```python
from build123d import *

# Parameters (mm, degrees)
F0_R        = 31.3722800925
F1_DEPTH    = 2.4
F0_R_2      = 27.0541255518
F2_DEPTH    = 14.1
F3_T1_DEPTH = 394.7097038856


# Not quite as in the source:
# - a fillet or chamfer that OpenCascade refuses, or shapes differently, is made with other operations: its cross-section is extruded or revolved along the edge and cut away or added


with BuildPart() as f1:
    # F0 (on Front) → F1 (new body)
    with BuildSketch(Plane.XZ):
        Polygon((76.1774070561, 60.170147568), (-76.1774070561, 60.170147568), (-76.1774070561, 34.1583490372), (-76.1774070561, -34.1583490372), (-76.1774070561, -60.170147568), (76.1774070561, -60.170147568), (76.1774070561, -34.1583490372), (76.1774070561, 34.1583490372), align=None)
        Circle(F0_R, mode=Mode.SUBTRACT)
    extrude(amount=F1_DEPTH)

    # F0 (on Front) → F2 (join)
    with BuildSketch(Plane.XZ):
        Circle(F0_R)
        Circle(F0_R_2, mode=Mode.SUBTRACT)
    extrude(amount=F2_DEPTH)

    # F3: fillet of radius 78.4619407771 on 4 edges, made by hand

    # F3_s2 → F3_t1 (cut)
    with BuildSketch(Plane.XZ.offset(-196.1548519428)):
        with BuildLine():
            ThreePointArc((2.284533721, 60.170147568), (-53.1964366675, 37.1891771794), (-76.1774070561, -18.2917932091))
            Line((-76.1774070561, -18.2917932091), (-76.1774070561, 60.170147568))
            Line((-76.1774070561, 60.170147568), (2.284533721, 60.170147568))
        make_face()
        with BuildLine():
            ThreePointArc((-2.284533721, 60.170147568), (53.1964366675, 37.1891771794), (76.1774070561, -18.2917932091))
            Line((76.1774070561, -18.2917932091), (76.1774070561, 60.170147568))
            Line((76.1774070561, 60.170147568), (-2.284533721, 60.170147568))
        make_face()
        with BuildLine():
            ThreePointArc((76.1774070561, 18.2917932091), (53.1964366675, -37.1891771794), (-2.284533721, -60.170147568))
            Line((-2.284533721, -60.170147568), (76.1774070561, -60.170147568))
            Line((76.1774070561, -60.170147568), (76.1774070561, 18.2917932091))
        make_face()
        with BuildLine():
            ThreePointArc((-76.1774070561, 18.2917932091), (-53.1964366675, -37.1891771794), (2.284533721, -60.170147568))
            Line((2.284533721, -60.170147568), (-76.1774070561, -60.170147568))
            Line((-76.1774070561, -60.170147568), (-76.1774070561, 18.2917932091))
        make_face()
    extrude(amount=F3_T1_DEPTH, mode=Mode.SUBTRACT)


solid = f1.part
```
CAD build for the part. Positions are in the model's coordinates, mm. A direction names the side the tool comes from. Round coordinates to 2 decimals unless told otherwise and drop trailing zeros. Loops run counter-clockwise (first coordinate to the right, second up) from the corner with the lowest first, then second, coordinate; pieces in that order, holes last. Notation, with made-up numbers: (-15, -1.75) - (-8, -1.75) arc R22 ccw to (-8, 15.25) - close; hole circle Ø11 at (81, 11). An arc over 180 degrees is marked (long way). Return JSON: item names as keys, results as strings. Group by question number.
Q1. Band-saw the part on B-B on x = 15. Give the cut face in (y, z).
Q2. Band-saw the part on D-D on z = -50.5. Give the cut face in (x, y).
Q3. Drill centre lines: line 1 along Z through (x, y) = (1, -6.75); line 2 along Y through (x, z) = (13.5, 43); line 3 along Z through (x, y) = (0, -6.75). Where is each one in solid material? Low to high. Write a range as [from, to].
Q4. Band-saw the part on A-A on z = -12. Give the cut face in (x, y), plus the area to 3 significant figures.
Q5. Tool access for faces 5 (the face through (-6.801, -8.168, -30.626)), 6 (the face through (-46.634, -1.183, 43.054)): list every direction of +Z, -Z, +X, -X, +Y, -Y with a clear straight run to the whole face (end or side of a thin tool).
Q6. Band-saw the part on C-C on y = -4.5. Give the cut face in (x, z), plus the area to 3 significant figures.
Q7. Two-plate mould, pull along Z, no slides. Class faces 1 (the face through (-26, -14.1, -9)), 2 (the face through (46.634, -1.183, 43.054)), 3 (the face through (25.805, -6.951, 8.126)), 4 (the face through (47.747, -1.183, -42.149)): +Z half, -Z half, draft (parallel to the pull), parting line (faces both ways), or undercut.
Q8. Flat gauge pins, fed straight in: pin 1 Ø1.5 at (y, z) = (-8.5, -26) entering from +X; pin 2 Ø5 at (x, y) = (-36.5, -2) entering from -Z; pin 3 Ø10 at (x, z) = (-49, -41.5) entering from +Y; pin 4 Ø1 at (x, y) = (-14.5, -10) entering from +Z. Where does each tip first touch, or does it go through?
Solutions:
{
 "1": {"outline": "(-14.1, -27.55) - (-2.4, -27.55) - (-2.4, -58.24) - (0, -58.24) - (0, -22.52) - (-14.1, -22.52) - close; (-14.1, 22.52) - (0, 22.52) - (0, 58.24) - (-2.4, 58.24) - (-2.4, 27.55) - (-14.1, 27.55) - close"},
 "2": {"outline": "(-35.45, -2.4) - (35.45, -2.4) - (35.45, 0) - (-35.45, 0) - close"},
 "3": {"line 1": "z = [-31.36, -27.04], [27.04, 31.36]", "line 2": "y = [-2.4, 0]", "line 3": "z = [-31.37, -27.05], [27.05, 31.37]"},
 "4": {"outline": "(-70.09, -2.4) - (-28.99, -2.4) - (-28.99, -14.1) - (-24.25, -14.1) - (-24.25, 0) - (-70.09, 0) - close; (24.25, -14.1) - (28.99, -14.1) - (28.99, -2.4) - (70.09, -2.4) - (70.09, 0) - (24.25, 0) - close", "area": "331 mm^2"},
 "5": {"face 5": "-Y", "face 6": "+Z, -X, +Y, -Y"},
 "6": {"outline": "circle Ø62.74 at (0, 0); hole circle Ø54.11 at (0, 0)", "area": "793 mm^2"},
 "7": {"face 1": "draft", "face 2": "+Z half", "face 3": "undercut", "face 4": "-Z half"},
 "8": {"pin 1": "stops at x = 18.62", "pin 2": "stops at z = -51.28", "pin 3": "stops at y = 0", "pin 4": "stops at z = 28.08"}
}
